The model under review builds one solid part; all positions refer to its coordinate system, in mm. A direction names the side the tool comes from. Round coordinates to 2 decimals unless told otherwise and drop trailing zeros. Order: outer loops, then holes, each group sorted by start corner. A loop starts at its lowest first (then second) coordinate and runs counter-clockwise, first axis right, second up. Notation, with made-up numbers: M -12,-23 L 32,-23 A16 ccw 32,-10 Z; hole C 55,-11 d11. An arc over 180 degrees is marked long. Use a Markdown table: item, result. Add a question column.
1. Consider section B-B on z = 11. State the section outline as (x, y) points, then the cut area to 3 significant figures.
2. Consider section D-D on z = 37.5. State the section outline as (x, y) points, then the cut area to 3 significant figures.
3. To check wall thickness, follow probe 1 along Z at (x, y) = (8.25, 5.5); probe 2 along Y at (x, z) = (0, 22); probe 3 along X at (y, z) = (-2, 35). State the ranges of each line that lie inside material, in increasing order.
4. The part is to be moulded in two halves that separate along Z. For faces 1 (the flat face through (9, -6.5, 19.4)), 2 (the flat face through (0, -7, 8)), say which applies: +Z half, -Z half, draft (parallel to the pull), parting line (faces both ways), or undercut.
5. Consider section A-A on x = 0. State the section outline as (y, z) points, then the cut area to 4 significant figures.
6. For faces 3 (the flat face through (-8, -0.1, 18.5)), 4 (the flat face through (9, 0, 18)), 5 (the cylindrical face through (-0.16, -7.01, 12.24)), list the 3-axis set-ups (+Z, -Z, +X, -X, +Y, -Y) from which the entire face can be reached by the end or side of a thin tool; tool diameter is ignored.
7. Consider section C-C on x = 8.75. State the section outline as (y, z) points, then the cut area to 3 significant figures.
from build123d import *

# Parameters (mm, degrees)
SKETCH1_W           = 20
SKETCH1_H           = 15
BOSS_EXTRUDE1_DEPTH = 45
SKETCH2_R           = 4
CUT_EXTRUDE1_DEPTH  = 46
CHAMFER1_SIZE       = 2
SKETCH4_W           = 2
SKETCH4_H           = 1
CUT_EXTRUDE2_DEPTH  = 16
SKETCH5_W           = 4
SKETCH5_H           = 8
SKETCH5_R           = 1.25
CUT_EXTRUDE3_DEPTH  = 1


with BuildPart() as part:
    # Sketch1 → Boss-Extrude1 (new body)
    with BuildSketch(Plane.XY):
        Rectangle(SKETCH1_W, SKETCH1_H)
    extrude(amount=BOSS_EXTRUDE1_DEPTH)

    # Sketch2 → Cut-Extrude1 (cut, through all)
    with BuildSketch(Plane.XY.offset(45)):
        Circle(SKETCH2_R)
    extrude(amount=-CUT_EXTRUDE1_DEPTH, mode=Mode.SUBTRACT)

    # Chamfer1
    chamfer1_edges = [part.edges().sort_by_distance(p)[0] for p in [
        (10, 7.5, 22.5),
        (10, -7.5, 22.5),
        (-10, -7.5, 22.5),
        (-10, 7.5, 22.5),
    ]]
    chamfer(chamfer1_edges, length=CHAMFER1_SIZE)

    # Sketch4 → Cut-Extrude2 (cut, through all)
    with BuildSketch(Plane.XZ.offset(7.5)):
        with Locations((-9, 15)):
            Rectangle(SKETCH4_W, SKETCH4_H)
        with Locations((-9, 16.75)):
            Rectangle(SKETCH4_W, SKETCH4_H)
        with Locations((-9, 18.5)):
            Rectangle(SKETCH4_W, SKETCH4_H)
        with Locations((-9, 20.25)):
            Rectangle(SKETCH4_W, SKETCH4_H)
        with Locations((-9, 22)):
            Rectangle(SKETCH4_W, SKETCH4_H)
        with Locations((9, 22)):
            Rectangle(SKETCH4_W, SKETCH4_H)
        with Locations((9, 20.25)):
            Rectangle(SKETCH4_W, SKETCH4_H)
        with Locations((9, 18.5)):
            Rectangle(SKETCH4_W, SKETCH4_H)
        with Locations((9, 16.75)):
            Rectangle(SKETCH4_W, SKETCH4_H)
        with Locations((9, 15)):
            Rectangle(SKETCH4_W, SKETCH4_H)
    extrude(amount=-CUT_EXTRUDE2_DEPTH, mode=Mode.SUBTRACT)

    # Sketch5 → Cut-Extrude3 (cut)
    with BuildSketch(Plane.XZ.offset(7.5)):
        with Locations((0, 12)):
            Rectangle(SKETCH5_W, SKETCH5_H)
        with Locations((0, 11)):
            Circle(SKETCH5_R, mode=Mode.SUBTRACT)
    extrude(amount=-CUT_EXTRUDE3_DEPTH, mode=Mode.SUBTRACT)


solid = part.part
Answer block:
| question | item | result |
|---|---|---|
| 1 | outline | M -10,-5.5 L -8,-7.5 L -2,-7.5 L -2,-6.5 L -1.25,-6.5 L -1.25,-7.5 L 1.25,-7.5 L 1.25,-6.5 L 2,-6.5 L 2,-7.5 L 8,-7.5 L 10,-5.5 L 10,5.5 L 8,7.5 L -8,7.5 L -10,5.5 Z; hole C 0,0 d8 |
| 1 | area | 240 mm^2 |
| 2 | outline | M -10,-5.5 L -8,-7.5 L 8,-7.5 L 10,-5.5 L 10,5.5 L 8,7.5 L -8,7.5 L -10,5.5 Z; hole C 0,0 d8 |
| 2 | area | 242 mm^2 |
| 3 | probe 1 | 0 to 14.5, 15.5 to 16.25, 17.25 to 18, 19 to 19.75, 20.75 to 21.5, 22.5 to 45 |
| 3 | probe 2 | -7.5 to -4, 4 to 7.5 |
| 3 | probe 3 | -10 to -3.46, 3.46 to 10 |
| 4 | face 1 | draft |
| 4 | face 2 | undercut |
| 5 | outline | M -7.5,0 L -4,0 L -4,45 L -7.5,45 L -7.5,16 L -6.5,16 L -6.5,12.25 L -7.5,12.25 L -7.5,9.75 L -6.5,9.75 L -6.5,8 L -7.5,8 Z; M 4,0 L 7.5,0 L 7.5,45 L 4,45 Z |
| 5 | area | 309.5 mm^2 |
| 6 | face 3 | -X, +Y, -Y |
| 6 | face 4 | +X, +Y, -Y |
| 6 | face 5 | -Y |
| 7 | outline | M -6.75,0 L 6.75,0 L 6.75,14.5 L -6.75,14.5 Z; M -6.75,15.5 L 6.75,15.5 L 6.75,16.25 L -6.75,16.25 Z; M -6.75,17.25 L 6.75,17.25 L 6.75,18 L -6.75,18 Z; M -6.75,19 L 6.75,19 L 6.75,19.75 L -6.75,19.75 Z; M -6.75,20.75 L 6.75,20.75 L 6.75,21.5 L -6.75,21.5 Z; M -6.75,22.5 L 6.75,22.5 L 6.75,45 L -6.75,45 Z |
| 7 | area | 540 mm^2 |
